Part model, mm, in its own coordinate system. A direction names the side the tool comes from. Give positions to 0.01 mm unless a question says otherwise; leave off trailing zeros. Write each loop counter-clockwise with the first axis right and the second up, starting at its lowest first coordinate (ties: lowest second). Pieces come first, ordered by that corner, then holes. Notation, with made-up numbers: M 29,51.5 L 58,51.5 A18 cw 58,72.5 Z; hole C 71,19.5 d2. An arc over 180 degrees is marked long. Use CSV: the item, a comma, the result in double quotes. Start each with the question number.
1. Band-saw the part on B-B, the plane x = 14. List the corners of the cut face in (y, z).
2. Band-saw the part on A-A, the plane z = 21. List the corners of the cut face in (x, y).
3. Drill centre lines: line 1 along Y through (x, z) = (31.75, 23); line 2 along Y through (x, z) = (38.5, 23.25); line 3 along Z through (x, y) = (54.5, 16). Where is each one in solid material? Low to high. Write a range as from..to.
4. Band-saw the part on C-C, the plane y = 22.5. List the corners of the cut face in (x, z), then the cut area to 3 significant figures.
5. 3-axis set-ups, long thin cutter, end or side, ignore diameter. For faces 3 (the face through (31, 32, 12.7)), 4 (the face through (31, 32, 0)): which of +Z, -Z, +X, -X, +Y, -Y reach the whole face in a straight line?
6. Drop flat-ended pins along their axis: pin 1 Ø1.5 at (x, y) = (19.5, 8.5) entering from +Z; pin 2 Ø1.5 at (x, z) = (16.5, 9) entering from +Y; pin 3 Ø12 at (y, z) = (18, 14.5) entering from -X. Give the stop position or say it passes through.
7. Mould opens along X. For faces 1 (the face through (27.98, 60.48, 19.14)), 2 (the face through (6, 46, 25.4)) say: pulls with the +X half, pulls with the -X half, needs draft (parallel to the pull), parting line crosses it, or undercut.
8. Band-saw the part on D-D, the plane z = 5.5. List the corners of the cut face in (x, y).
from build123d import *

# Parameters (mm, degrees)
F0_W     = 63.5
F0_H     = 63.5
F1_DEPTH = 25.4
F3_DEPTH = 25.4
F4_R     = 28.974598
F5_DEPTH = 12.7


with BuildPart() as f1:
    # F0 (on Top) → F1 (new body)
    with BuildSketch(Plane.XY):
        with Locations((31.75, 31.75)):
            Rectangle(F0_W, F0_H)
    extrude(amount=F1_DEPTH)

    # F2 (on face) → F3 (cut)
    with BuildSketch(Plane.XY.offset(25.4)):
        with BuildLine():
            Line((31.75, 62.834862), (31.75, 63.5))
            Line((31.75, 63.5), (0, 63.5))
            Line((0, 63.5), (0, 31.75))
            Line((0, 31.75), (0.665138, 31.75))
            ThreePointArc((0.665138, 31.75), (9.769684, 53.730316), (31.75, 62.834862))
        make_face()
        with BuildLine():
            Line((63.5, 63.5), (31.75, 63.5))
            Line((31.75, 63.5), (31.75, 62.834862))
            ThreePointArc((31.75, 62.834862), (53.730316, 53.730316), (62.834862, 31.75))
            Line((62.834862, 31.75), (63.5, 31.75))
            Line((63.5, 31.75), (63.5, 63.5))
        make_face()
        with BuildLine():
            Line((63.5, 31.75), (62.834862, 31.75))
            ThreePointArc((62.834862, 31.75), (53.730316, 9.769684), (31.75, 0.665138))
            Line((31.75, 0.665138), (31.75, 0))
            Line((31.75, 0), (63.5, 0))
            Line((63.5, 0), (63.5, 31.75))
        make_face()
        with BuildLine():
            ThreePointArc((31.75, 0.665138), (9.769684, 9.769684), (0.665138, 31.75))
            Line((0.665138, 31.75), (0, 31.75))
            Line((0, 31.75), (0, 0))
            Line((0, 0), (31.75, 0))
            Line((31.75, 0), (31.75, 0.665138))
        make_face()
    extrude(amount=-F3_DEPTH, mode=Mode.SUBTRACT)

    # F4 (on face) → F5 (cut)
    with BuildSketch(Plane.XY.offset(25.4)):
        with Locations((31.75, 31.75)):
            Circle(F4_R)
    extrude(amount=-F5_DEPTH, mode=Mode.SUBTRACT)


solid = f1.part
Output:
1,outline,"M 6.23,0 L 57.27,0 L 57.27,25.4 L 54.65,25.4 L 54.65,12.7 L 8.85,12.7 L 8.85,25.4 L 6.23,25.4 Z"
2,outline,"M 0.67,31.75 A31.08 ccw 31.75,0.67 A31.08 ccw 62.83,31.75 A31.08 ccw 31.75,62.83 A31.08 ccw Z; hole C 31.75,31.75 d57.95"
3,line 1,"y = 0.67..2.78, 60.72..62.83"
3,line 2,"y = 1.41..3.57, 59.93..62.09"
3,line 3,"z = 0..12.7"
4,outline,"M 2.07,0 L 61.43,0 L 61.43,25.4 L 59.21,25.4 L 59.21,12.7 L 4.29,12.7 L 4.29,25.4 L 2.07,25.4 Z"
4,area,"810 mm²"
5,face 3,"+Z"
5,face 4,"-Z, +X, -X, +Y, -Y"
6,pin 1,"stops at z = 12.7"
6,pin 2,"stops at y = 59.25"
6,pin 3,"stops at x = 1.65"
7,face 1,"undercut"
7,face 2,"needs draft"
8,outline,"M 0.67,31.75 A31.08 ccw 31.75,0.67 A31.08 ccw 62.83,31.75 A31.08 ccw 31.75,62.83 A31.08 ccw Z"
